Study the drawing (mm; zero at the part's minimum x, y, z) and answer. A direction names the side the tool comes from. Give positions to 0.01 mm unless a question says otherwise; leave off trailing zeros. Write each loop counter-clockwise with the first axis right and the second up, starting at its lowest first coordinate (ties: lowest second). Pieces come first, ordered by that corner, then holes.
1) Straight lines are drawn through the part: probe 1 along X at (y, z) = (4.5, 3.55); probe 2 along Z at (x, y) = (1.3, 3.5); probe 3 along X at (y, z) = (11, 4). For each, find the intervals that lie inside material, in ascending order.
2) Find section C-C (y = 4.5). Determine the outline of the cut face in (x, z).
3) Determine the mould class of the marked faces 1, 2 and 3 for opening direction Y: pulls with the +Y half, pulls with the -Y half, needs draft (parallel to the pull), parting line crosses it, or undercut.
4) Find section D-D (z = 0.5). Count the separate pieces of the cut face and the enclosed holes in it, plus the area to 3 significant figures.
5) Given pin 1 Ø3 at (y, z) = (6, 4.5) entering from -X; pin 2 Ø2 at (x, y) = (4, 7.5) entering from +Z; pin 3 Ø1 at (x, y) = (4, 5) entering from -Z, each flat-ended and moving along its own axis, determine where each tip first touches the part or whether it passes through.
6) A tool of negligible diameter and unlimited length cuts with its end or side. For the marked faces 4 and 5, from which of +Z, -Z, +X, -X, +Y, -Y can it reach the whole face along a straight path? Write none if from no direction.
7) Find section A-A (x = 2.5). Determine the outline of the cut face in (y, z), plus the area to 3 significant figures.
8) Find section B-B (z = 2.5). Determine the outline of the cut face in (x, y).
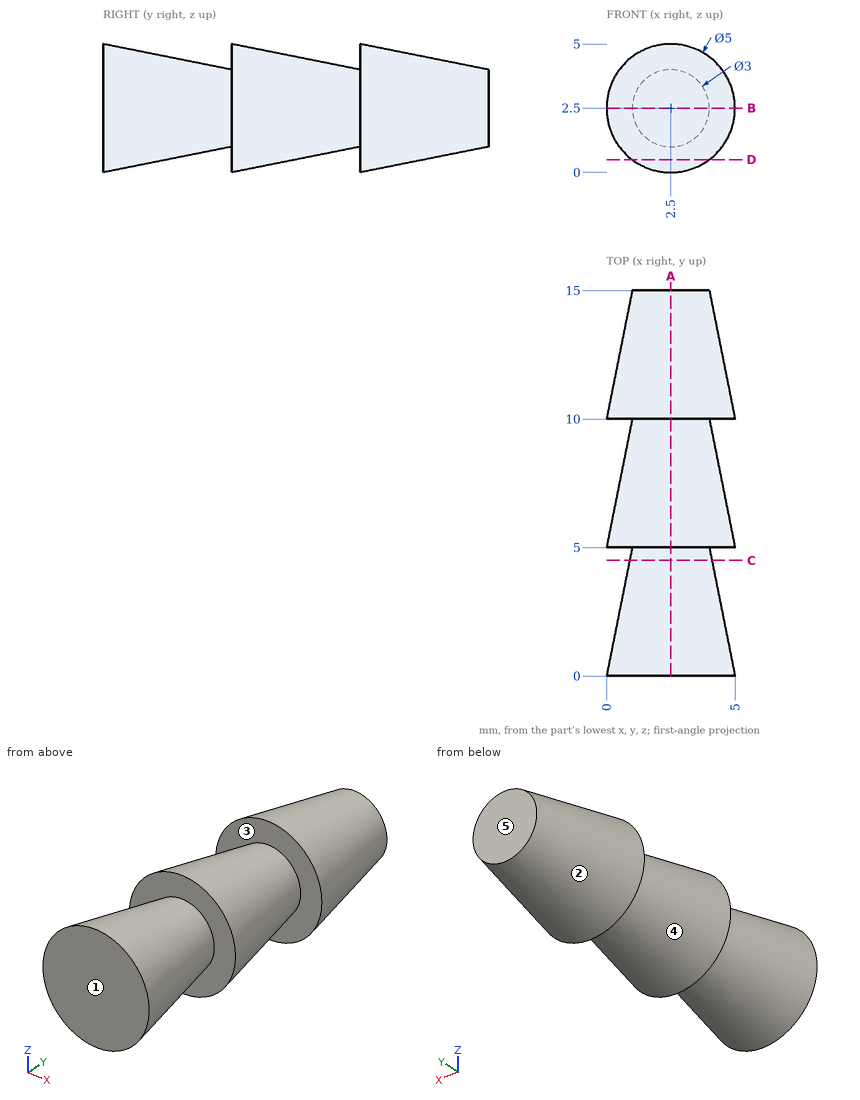
Results:
1. probe 1: x = 1.29 to 3.71
1. probe 2: z = 1.16 to 3.84
1. probe 3: x = 0.76 to 4.24
2. outline: circle Ø3.2 at (2.5, 2.5)
3. face 1: pulls with the -Y half
3. face 2: pulls with the +Y half
3. face 3: undercut
4. separate pieces: 3
4. enclosed holes: 0
4. area: 14.7 mm2
5. pin 1: stops at x = 0.15
5. pin 2: stops at z = 4.5
5. pin 3: stops at z = 0.21
6. face 4: none
6. face 5: +Z, -Z, +X, -X, +Y
7. outline: (0, 0) - (5, 1) - (5, 0) - (10, 1) - (10, 0) - (15, 1) - (15, 4) - (10, 5) - (10, 4) - (5, 5) - (5, 4) - (0, 5) - close
7. area: 60.0 mm2
8. outline: (0, 0) - (5, 0) - (4, 5) - (5, 5) - (4, 10) - (5, 10) - (4, 15) - (1, 15) - (0, 10) - (1, 10) - (0, 5) - (1, 5) - close
